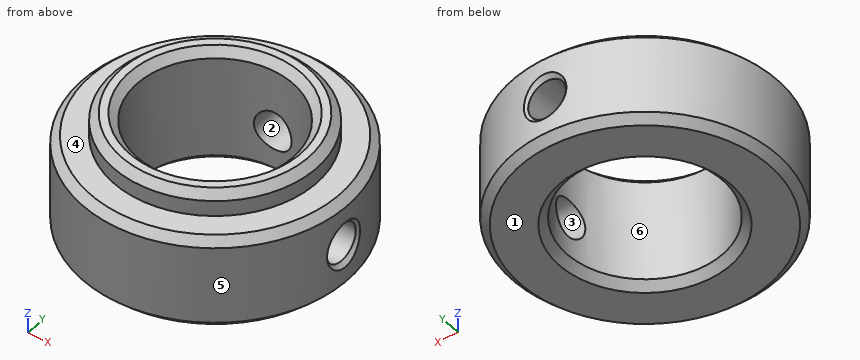
Autodesk Inventor part; units mm, degrees
ref_plane "body_set_h_XY" through (0, 8.5, 0) normal (0, 1, 0) x (1, 0, 0)
ref_plane "body_set_h_YZ" through (0, 8.5, 0) normal (1, 0, 0) x (0, 0, -1)
ref_plane "body_set_h_ZX" through (0, 8.5, 0) normal (0, 0, -1) x (0, 1, 0)
sketch "Sketch_1" plane through (0, 0, 0) normal (0, 1, 0) x (-1, 0, 0)
  line L0 (0, 4.5) -> (0, -3)
  line L1 (-5, 4) -> (-5.5, 4.5)
  line L2 (-5.5, 4.5) -> (-6, 4.5)
  line L3 (-6, 4.5) -> (-6.5, 4)
  line L4 (-6.5, 4) -> (-6.5, 3)
  line L5 (-6.5, 3) -> (-8, 3)
  line L6 (-8, 3) -> (-8.5, 2.5)
  line L7 (-8.5, 2.5) -> (-8.5, -2.5)
  line L8 (-8.5, -2.5) -> (-8, -3)
  line L9 (-8, -3) -> (-5.5, -3)
  line L10 (-5.5, -3) -> (-5, -2.5)
  line L11 (-5, -2.5) -> (-5, 4)
revolve "Revolution1" add sketch "Sketch_1" angle 360 about axis through (0, 0, 4.5) along (0, 0, -1)
sketch "Sketch_8" plane through (0, 0, 0) normal (0, 0, 1) x (1, 0, 0)
  line L0 (8.5, 0) -> (4, 0)
  line L1 (4, 0) -> (4, 1.2295)
  line L2 (4, 1.2295) -> (8.2295, 1.2295)
  line L3 (8.2295, 1.2295) -> (8.5, 1.5)
  line L4 (8.5, 1.5) -> (8.5, 0)
  line L5 (8.5, 0) -> (4, 0)
revolve "Revolution2" cut sketch "Sketch_8" angle 360 about axis through (8.5, 0, 0) along (-1, 0, 0)
thread "Thread1"
sketch "Sketch_2" plane through (0, 0, 0) normal (0, 0, 1) x (1, 0, 0)
  line L0 (0, 8.5) -> (0, 4)
  line L1 (0, 4) -> (-1.2295, 4)
  line L2 (-1.2295, 4) -> (-1.2295, 8.2295)
  line L3 (-1.2295, 8.2295) -> (-1.5, 8.5)
  line L4 (-1.5, 8.5) -> (0, 8.5)
  line L5 (0, 8.5) -> (0, 4)
revolve "Revolution3" cut sketch "Sketch_2" angle 360 about axis through (0, 8.5, 0) along (0, -1, 0)
thread "Thread2"
ref_plane "body_set_h_XY" through (0, 8.5, 0) normal (0, 1, 0) x (1, 0, 0)
ref_plane "body_set_h_YZ" through (0, 8.5, 0) normal (1, 0, 0) x (0, 0, -1)
ref_plane "body_set_h_ZX" through (0, 8.5, 0) normal (0, 0, -1) x (0, 1, 0)
ref_plane "body_set_v_XY" through (8.5, 0, 0) normal (1, 0, 0) x (0, 0, -1)
ref_plane "body_set_v_YZ" through (8.5, 0, 0) normal (0, 0, -1) x (0, 1, 0)
ref_plane "body_set_v_ZX" through (8.5, 0, 0) normal (0, 1, 0) x (1, 0, 0)
properties part number "SCBRJ10-13_b"
Verification items for the finished model (mm, model axes). Face numbers are marked on the shaded views. A direction names the side the tool comes from. Round coordinates to 2 decimals unless told otherwise and drop trailing zeros. Write each loop counter-clockwise with the first axis right and the second up, starting at its lowest first coordinate (ties: lowest second). Pieces come first, ordered by that corner, then holes.
1. Section check A-A on y = 0. Enter the section's corners in (x, z).
2. Scan lines: L1, parallel to Z at x = 0, y = 5.55; L2, parallel to Z at x = 6.7, y = 0; L3, parallel to Y at x = 0, z = -0.25. Record each from-to range of solid material in increasing order.
3. Gauge pin test, flat ends, axial feed: P1, Ø4, axis at y = 3, z = -1, coming from the +X side; P2, Ø3, axis at x = -3.5, z = 0, coming from the -Y side; P3, Ø6, axis at x = -5.5, y = 6, coming from the -Z side; P4, Ø4, axis at y = 6, z = 0.5, coming from the +X side. Record the tip position at first contact, or that the pin passes through.
4. Draft check along Y on the marked faces 3, 4, 5 and 6. Enter one of: +Y half, -Y half, draft (parallel to the pull), parting line (faces both ways), or undercut.
5. Section check D-D on z = 3.5. Enter the section's corners in (x, y), plus the area to 3 significant figures.
6. Section check C-C on z = 0. Enter the section's corners in (x, y).
7. Access from +Z, -Z, +X, -X, +Y, -Y to the whole of each face (thin tool, end or side, straight path). Record for the marked faces 1 and 2.
Answer:
1. outline: (-8.5, -2.5) - (-8, -3) - (-5.5, -3) - (-5, -2.5) - (-5, 4) - (-5.5, 4.5) - (-6, 4.5) - (-6.5, 4) - (-6.5, 3) - (-8, 3) - (-8.5, 2.5) - close; (5, -2.5) - (5.5, -3) - (8, -3) - (8.5, -2.5) - (8.5, -1.5) - (8.23, -1.23) - (5, -1.23) - close; (5, 1.23) - (8.23, 1.23) - (8.5, 1.5) - (8.5, 2.5) - (8, 3) - (6.5, 3) - (6.5, 4) - (6, 4.5) - (5.5, 4.5) - (5, 4) - close
2. L1: z = -3 to -1.23, 1.23 to 4.5
2. L2: z = -3 to -1.23, 1.23 to 3
2. L3: y = -8.5 to -5
3. P1: stops at x = 8.44
3. P2: stops at y = -8.26
3. P3: stops at z = -3
3. P4: stops at x = 7.5
4. face 3: undercut
4. face 4: draft
4. face 5: parting line
4. face 6: undercut
5. outline: circle Ø13 at (0, 0); hole circle Ø10 at (0, 0)
5. area: 54.2 mm2
6. outline: (-1.39, 8.39) arc R8.5 ccw (long way) to (8.39, -1.39) - (8.23, -1.23) - (4.85, -1.23) arc R5 cw (long way) to (-1.23, 4.85) - (-1.23, 8.23) - close; (1.23, 4.85) arc R5 cw to (4.85, 1.23) - (8.23, 1.23) - (8.39, 1.39) arc R8.5 ccw to (1.39, 8.39) - (1.23, 8.23) - close
7. face 1: -Z, +X, -X, +Y, -Y
7. face 2: +Y
